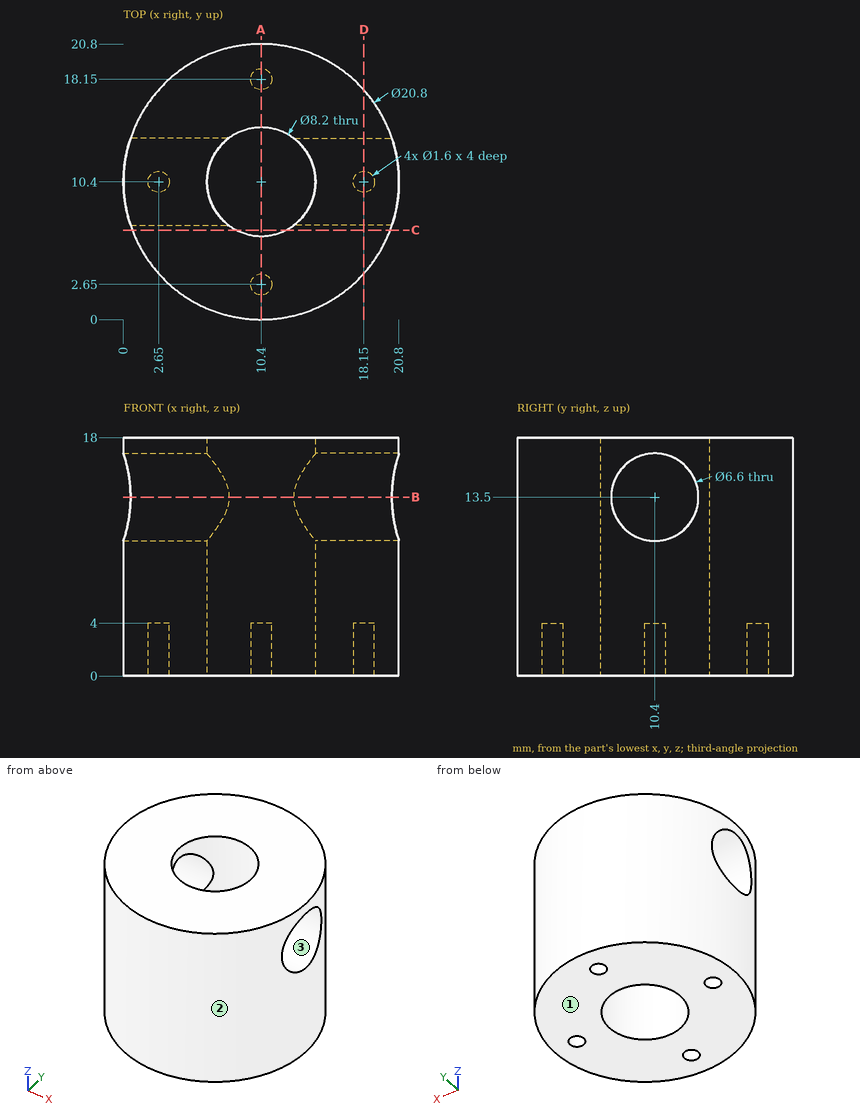
Geometry: see drawing. Coordinates: mm, zero at the bounding-box minimum. Give positions to 0.01 mm unless a question says otherwise; leave off trailing zeros. Loops run counter-clockwise (first coordinate to the right, second up) from the corner with the lowest first, then second, coordinate; pieces in that order, holes last. Notation, with made-up numbers: (-7, 9.5) - (42, 9.5) arc R8 ccw to (42, 18.5) - close; hole circle Ø5 at (71, 60). An arc over 180 degrees is marked (long way). Use CSV: the item, a comma, the result in double quotes.
1) Mould query, pull axis Y, two halves, no side actions, for the marked faces 1, 2 and 3. Classes: +Y half, -Y half, draft (parallel to the pull), parting line (faces both ways), or undercut.
Worked out:
face 1,"draft"
face 2,"parting line"
face 3,"undercut"
2) Cut plane C-C (y = 6.75). Output: boundary loops of the cut face in (x, z).
Worked out:
outline,"(0.66, 0) - (8.53, 0) - (8.53, 18) - (0.66, 18) - close; (12.27, 0) - (20.14, 0) - (20.14, 18) - (12.27, 18) - close"
3) Pin query (flat end, axial travel): P1, Ø10, axis at x = 9.5, z = 12.5, coming from the +Y side; P2, Ø3, axis at y = 17, z = 10, coming from the +X side; P3, Ø10, axis at x = 18.5, z = 14, coming from the +Y side; P4, Ø1, axis at x = 18.15, y = 10.4, coming from the -Z side. Return the tip coordinate at first contact, or that it passes through.
Worked out:
P1,"stops at y = 20.8"
P2,"stops at x = 19.46"
P3,"stops at y = 20.33"
P4,"stops at z = 4"
4) Cut plane B-B (z = 13.5). Output: boundary loops of the cut face in (x, y), and give its area (3 significant figures).
Worked out:
outline,"(0.54, 7.1) arc R10.4 ccw to (20.26, 7.1) - (12.83, 7.1) arc R4.1 cw to (7.97, 7.1) - close; (0.54, 13.7) - (7.97, 13.7) arc R4.1 cw to (12.83, 13.7) - (20.26, 13.7) arc R10.4 ccw to start"
area,"200 mm^2"
5) Line query: line 1 (Y direction, x = 10.4, z = 1.1); line 2 (X direction, y = 10.5, z = 8.75); line 3 (X direction, y = 13.75, z = 12.5). Output: solid intervals per line, ascending.
Worked out:
line 1,"y = 0 to 1.85, 3.45 to 6.3, 14.5 to 17.35, 18.95 to 20.8"
line 2,"x = 0 to 6.3, 14.5 to 20.8"
line 3,"x = 0.55 to 8.04, 12.76 to 20.25"
6) Cut plane D-D (x = 18.15). Output: boundary loops of the cut face in (y, z), and give its area (3 significant figures).
Worked out:
outline,"(3.46, 0) - (9.6, 0) - (9.6, 4) - (11.2, 4) - (11.2, 0) - (17.34, 0) - (17.34, 18) - (3.46, 18) - close; hole circle Ø6.6 at (10.4, 13.5)"
area,"209 mm^2"
7) Cut plane A-A (x = 10.4). Output: boundary loops of the cut face in (y, z), and give its area (3 significant figures).
Worked out:
outline,"(0, 0) - (1.85, 0) - (1.85, 4) - (3.45, 4) - (3.45, 0) - (6.3, 0) - (6.3, 18) - (0, 18) - close; (14.5, 0) - (17.35, 0) - (17.35, 4) - (18.95, 4) - (18.95, 0) - (20.8, 0) - (20.8, 18) - (14.5, 18) - close"
area,"214 mm^2"
